Autodesk Fusion 360 part; units mm, degrees
sketch "Skizze1" plane through (0, 0, 0) normal (0, 1, 0) x (1, 0, 0)
  line L0 (5, 0) -> (2.5, 4.3301)
  line L1 (2.5, 4.3301) -> (-2.5, 4.3301)
  line L2 (-2.5, 4.3301) -> (-5, 0)
  line L3 (-5, 0) -> (-2.5, -4.3301)
  line L4 (-2.5, -4.3301) -> (2.5, -4.3301)
  line L5 (2.5, -4.3301) -> (5, 0)
  circle A0 centre (0, 0) radius 3.55
  circle A1 centre (0, 0.828) radius 2.6
  dimension "d1" = 10
  dimension "d2" = 7.1
  dimension "d3" = 5.2
extrude "Extrusion1" add sketch "Skizze1" along normal blind 8.4 contours L0 L1 L2 L3 L4 L5 | A0
extrude "Extrusion2" add sketch "Skizze1" along normal blind 2.5 from surface at 8.4 contours A0
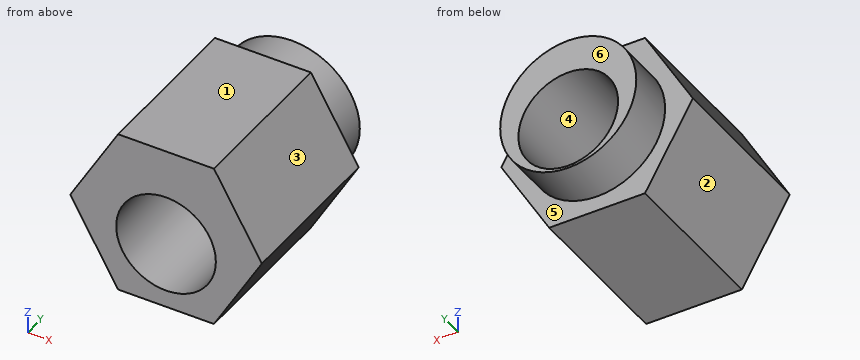
Input: part model. Units: mm. Frame: model coordinates. Face numbers are marked on the shaded views. A direction names the side the tool comes from. Give positions to 0.01 mm unless a question says otherwise; leave off trailing zeros. Order: outer loops, then holes, each group sorted by start corner. A loop starts at its lowest first (then second) coordinate and runs counter-clockwise, first axis right, second up.
1. Mould query, pull axis X, two halves, no side actions, for the marked faces 1, 2, 3 and 4. Classes: released by +X, released by -X, zero draft, split by the parting line, or undercut.
Derived:
face 1: zero draft
face 2: released by -X
face 3: released by +X
face 4: undercut
2. Material intervals for L1, parallel to Z at x = 0, y = 8.25; L2, parallel to Z at x = 2.25, y = 3.5; L3, parallel to X at y = 3.75, z = -1.5, sorted ascending.
Derived:
L1: z = -4.33 to -3.43, 1.77 to 4.33
L2: z = -4.33 to -2.13, 0.47 to 4.33
L3: x = -4.13 to -2.51, 2.51 to 4.13
3. Section D-D on x = 4.25. Return the cut outline in (y, z), and give its area (3 significant figures).
Derived:
outline: (0, -1.3) - (8.4, -1.3) - (8.4, 1.3) - (0, 1.3) - close
area: 21.8 mm2
4. Section C-C on y = 5. Return the cut outline in (x, z).
Derived:
outline: (-5, 0) - (-2.5, -4.33) - (2.5, -4.33) - (5, 0) - (2.5, 4.33) - (-2.5, 4.33) - close; hole circle Ø5.2 at (0, -0.83)
5. Section A-A on x = 0. Return the cut outline in (y, z), and give its area (3 significant figures).
Derived:
outline: (0, -4.33) - (8.4, -4.33) - (8.4, -3.55) - (10.9, -3.55) - (10.9, -3.43) - (0, -3.43) - close; (0, 1.77) - (10.9, 1.77) - (10.9, 3.55) - (8.4, 3.55) - (8.4, 4.33) - (0, 4.33) - close
area: 33.8 mm2
6. Reachability of the marked faces 5 and 6 from +Z, -Z, +X, -X, +Y, -Y: full face, straight path, thin tool, end or side. Return the list, or none.
Derived:
face 5: +Y
face 6: +Z, -Z, +X, -X, +Y
7. Section B-B on z = -1.25. Return the cut outline in (x, y).
Derived:
outline: (-4.28, 0) - (-2.57, 0) - (-2.57, 10.9) - (-3.32, 10.9) - (-3.32, 8.4) - (-4.28, 8.4) - close; (2.57, 0) - (4.28, 0) - (4.28, 8.4) - (3.32, 8.4) - (3.32, 10.9) - (2.57, 10.9) - close
8. Pin query (flat end, axial travel): pin 1 (1.5 mm diameter, centred on x = -1.5, z = 1, fed in from -Y); pin 2 (5 mm diameter, centred on y = 4, z = 3.5, fed in from -X). Return the tip coordinate at first contact, or that it passes through.
Derived:
pin 1: stops at y = 0
pin 2: stops at x = -4.42
